Design review of the part shown in the three views and the two pictorial views. Dimensions are in mm from the part's minimum x, y and z. Coordinates: 2 decimals unless noted, no trailing zeros. Loops run counter-clockwise (first coordinate to the right, second up) from the corner with the lowest first, then second, coordinate; pieces in that order, holes last. Notation, with made-up numbers: M 6.5,-8.5 L 48.5,-8.5 A20 cw 48.5,-2.5 Z; hole C 42,27 d2. An arc over 180 degrees is marked long. Use CSV: the item, a comma, the result in double quotes. Start each with the question number.
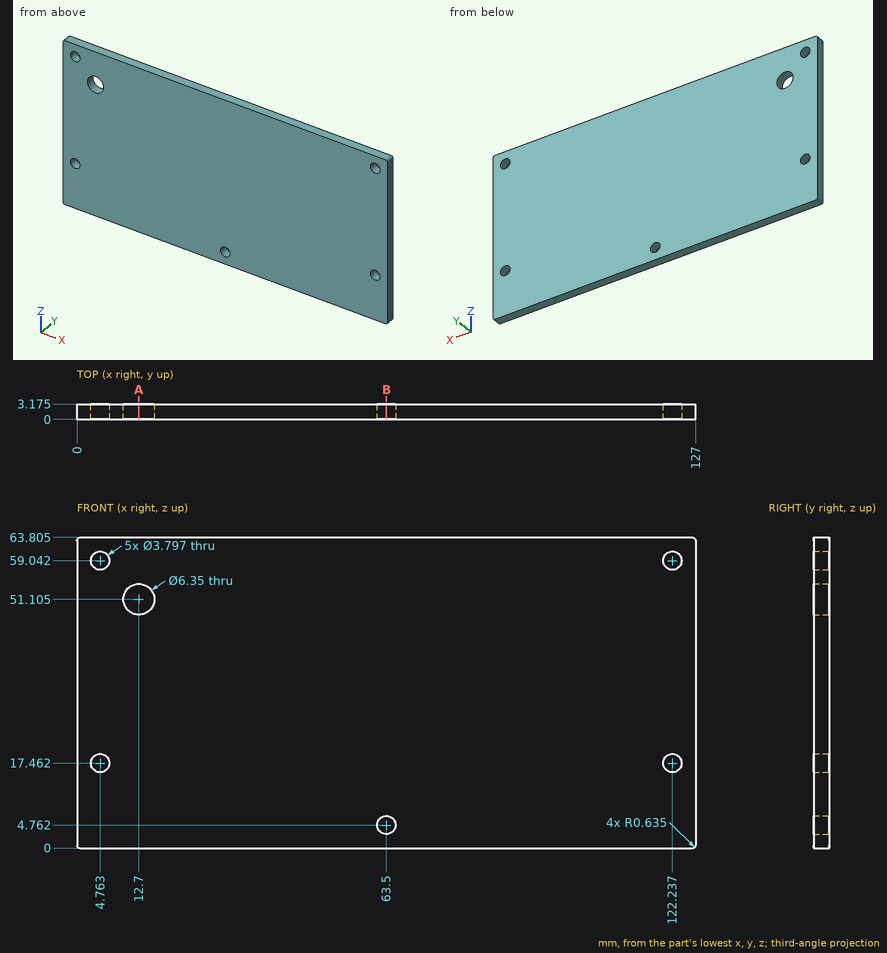
1. Add section A-A (x = 12.7). Write out the cut boundary in (y, z) (1 decimal).
2. To check wall thickness, follow line 1 along Z through (x, y) = (6, 0.8) (1 decimal); line 2 along X through (y, z) = (2.8, 51); line 3 along Z through (x, y) = (12.7, 1.9) (1 decimal). State the ranges of each line that lie inside material, in increasing order.
3. Insertion check: pin 1 Ø4 at (x, z) = (12.7, 51.1) entering from +Y. The pin has a flat end and moves straight along its axis. Give the tip position at first contact, or say it passes through.
4. Add section B-B (x = 63.5). Write out the cut boundary in (y, z) (1 decimal).
Solved:
1,outline,"M 0,0 L 3.2,0 L 3.2,47.9 L 0,47.9 Z; M 0,54.3 L 3.2,54.3 L 3.2,63.8 L 0,63.8 Z"
2,line 1,"z = 0 to 16, 18.9 to 57.6, 60.5 to 63.8"
2,line 2,"x = 0 to 9.53, 15.87 to 127"
2,line 3,"z = 0 to 47.9, 54.3 to 63.8"
3,pin 1,"passes through"
4,outline,"M 0,0 L 3.2,0 L 3.2,2.9 L 0,2.9 Z; M 0,6.7 L 3.2,6.7 L 3.2,63.8 L 0,63.8 Z"
